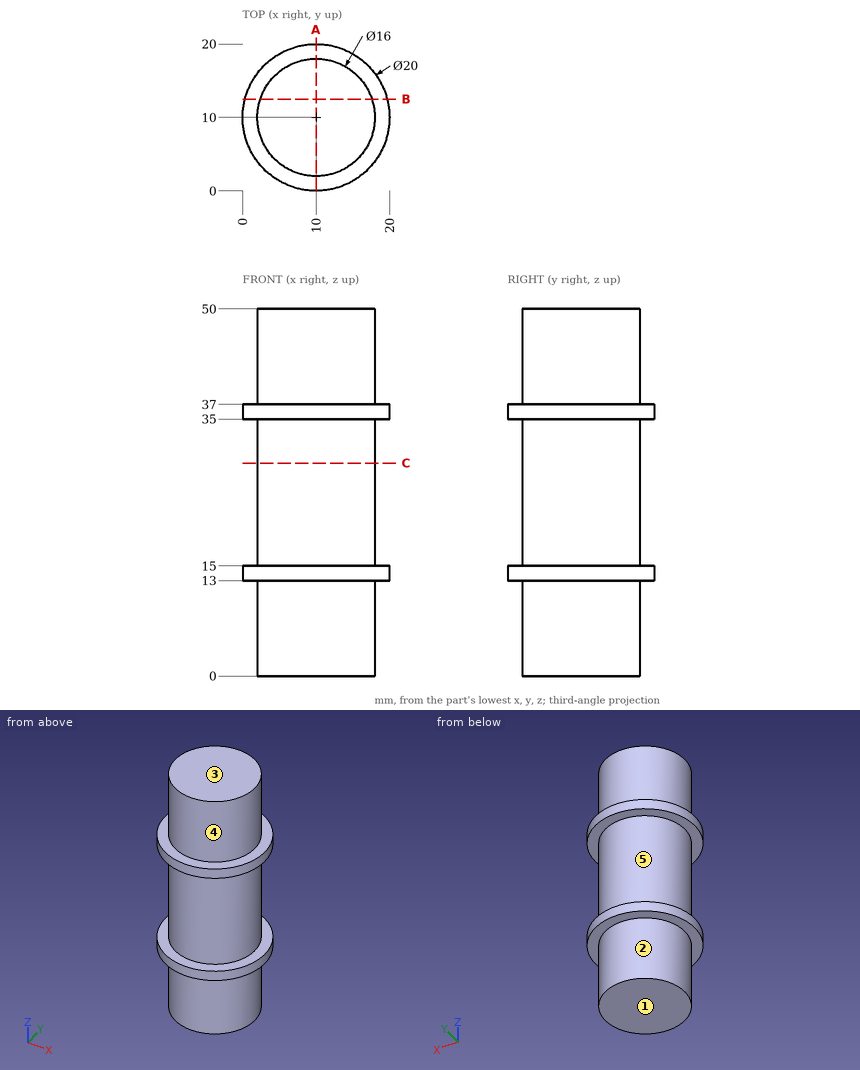
Can you work these out from the drawing? Everything is in mm from the part's minimum corner. A direction names the side the tool comes from. Give positions to 0.01 mm unless a question says otherwise; leave off trailing zeros. Loops run counter-clockwise (first coordinate to the right, second up) from the corner with the lowest first, then second, coordinate; pieces in that order, holes last. Notation, with made-up numbers: (75.5, -1) -> (129.5, -1) arc R23 cw to (129.5, 13) -> close; hole circle Ø6 at (64.25, -14.75). An arc over 180 degrees is marked (long way). Write item = value, one per line.
1) Suppose I cut it at C-C on z = 29. Write out the boundary of the cut face in (x, y), then the cut area to 3 significant figures.
Check result:
outline = circle Ø16 at (10, 10)
area = 201 mm2
2) Suppose I cut it at A-A on x = 10. Write out the boundary of the cut face in (y, z).
Check result:
outline = (0, 13) -> (2, 13) -> (2, 0) -> (18, 0) -> (18, 13) -> (20, 13) -> (20, 15) -> (18, 15) -> (18, 35) -> (20, 35) -> (20, 37) -> (18, 37) -> (18, 50) -> (2, 50) -> (2, 37) -> (0, 37) -> (0, 35) -> (2, 35) -> (2, 15) -> (0, 15) -> close
3) Will these pins go through, and if not, where does the flat tip stop? pin 1 (10 mm diameter, centred on x = 11, z = 26.5, fed in from -Y); pin 2 (5 mm diameter, centred on y = 7, z = 36.5, fed in from +X); pin 3 (10 mm diameter, centred on x = 14.5, z = 42.5, fed in from +Y).
Check result:
pin_1 = 2
pin_2 = 19.99
pin_3 = 18
4) For the marked faces 1 and 2, which set-ups out of +Z, -Z, +X, -X, +Y, -Y let a thin tool reach every point of the face, with its end or its side?
Check result:
face_1 = -Z, +X, -X, +Y, -Y
face_2 = -Z
5) I need wall thicknesses on L1, parallel to Z at x = 18.5, y = 6; L2, parallel to Y at x = 9.75, z = 29; L3, parallel to Y at x = 17.25, z = 22.5. Which ranges of each line are inside material? Lowest first, please. Write a range as from..to.
Check result:
L1 = 13..15, 35..37
L2 = 2..18
L3 = 6.62..13.38
6) Thinking about a two-plate mould opening in Z: for the marked faces 3, 4 and 5, which applies, released by +Z, released by -Z, zero draft, split by the parting line, or undercut?
Check result:
face_3 = released by +Z
face_4 = zero draft
face_5 = undercut
7) Suppose I cut it at B-B on y = 12.5. Write out the boundary of the cut face in (x, z).
Check result:
outline = (0.32, 13) -> (2.4, 13) -> (2.4, 0) -> (17.6, 0) -> (17.6, 13) -> (19.68, 13) -> (19.68, 15) -> (17.6, 15) -> (17.6, 35) -> (19.68, 35) -> (19.68, 37) -> (17.6, 37) -> (17.6, 50) -> (2.4, 50) -> (2.4, 37) -> (0.32, 37) -> (0.32, 35) -> (2.4, 35) -> (2.4, 15) -> (0.32, 15) -> close
